Drawing for the job (mm, zero at the part's lowest x, y, z). A direction names the side the tool comes from. Give positions to 0.01 mm unless a question says otherwise; leave off trailing zeros. Order: outer loops, then holes, each group sorted by start corner. A loop starts at its lowest first (then second) coordinate and runs counter-clockwise, first axis right, second up. Notation, with made-up numbers: (25.25, 80) - (36.25, 80) arc R31 cw to (36.25, 119) - close; hole circle Ø9 at (19, -5). An arc over 180 degrees is marked (long way). One line per item, written item: value.
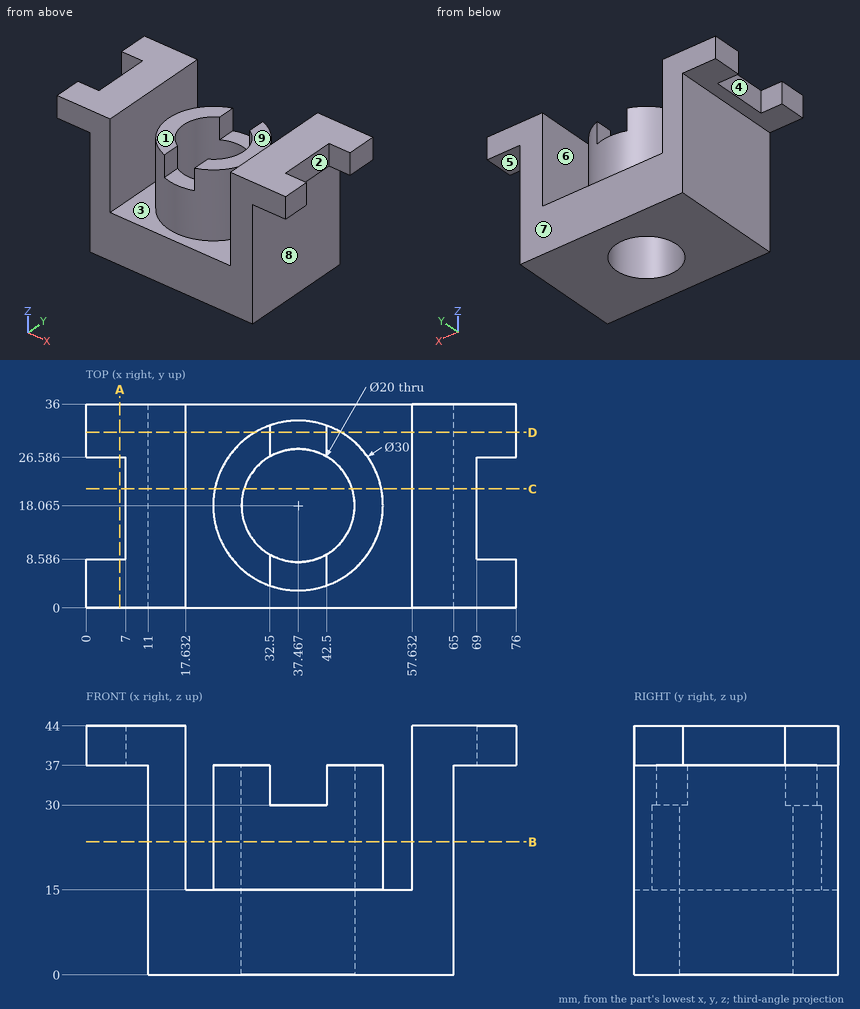
1) Cut at B-B, the plane z = 23.5. Give the cut face in (x, y) (1 decimal).
Outcome:
outline: (11, 0) - (17.6, 0) - (17.6, 36) - (11, 36) - close; circle Ø30 at (37.5, 18.1); (57.6, 0) - (65, 0) - (65, 36) - (57.6, 36) - close; hole circle Ø20 at (37.5, 18.1)
2) Drill centre lines: line 1 along Y through (x, z) = (38, 7); line 2 along X through (y, z) = (13.5, 19.5) (1 decimal); line 3 along X through (y, z) = (21.5, 29.5) (1 decimal). Where is each one in solid material? Low to high. Write a range as from..to.
Outcome:
line 1: y = 0..8.08, 28.05..36
line 2: x = 11..17.6, 23.2..28.6, 46.4..51.8, 57.6..65
line 3: x = 11..17.6, 22.9..28.1, 46.9..52.1, 57.6..65
3) Cut at A-A, the plane x = 6. Give the cut face in (y, z) (1 decimal).
Outcome:
outline: (0, 37) - (8.6, 37) - (8.6, 44) - (0, 44) - close; (26.6, 37) - (36, 37) - (36, 44) - (26.6, 44) - close
4) Which spindle directions (+Z, -Z, +X, -X, +Y, -Y) get a long thin tool onto all of the face, cutting with end or side? Do the marked faces 1, 2, 3, 4 and 5. Say none if no direction does.
Outcome:
face 1: +Z, +Y, -Y
face 2: +Z, -Z, +X
face 3: +Z
face 4: +Z, -Z, -X
face 5: -Z, +X, +Y, -Y
5) Pin check, flat tips, straight feed: pin 1 (12 mm diameter, centred on x = 4.5, y = 14.5, fed in from -Z); pin 2 (11 mm diameter, centred on x = 26, y = 19, fed in from +Z); pin 3 (1.9 mm diameter, centred on x = 35.5, y = 29.5, fed in from +Z). Stop position of each tip, or through.
Outcome:
pin 1: stops at z = 37
pin 2: stops at z = 37
pin 3: stops at z = 30
6) Cut at D-D, the plane y = 31. Give the cut face in (x, z).
Outcome:
outline: (0, 37) - (11, 37) - (11, 0) - (65, 0) - (65, 37) - (76, 37) - (76, 44) - (57.63, 44) - (57.63, 15) - (45.06, 15) - (45.06, 37) - (42.5, 37) - (42.5, 30) - (32.5, 30) - (32.5, 37) - (29.87, 37) - (29.87, 15) - (17.63, 15) - (17.63, 44) - (0, 44) - close
7) Cut at C-C, the plane y = 21. Give the cut face in (x, z).
Outcome:
outline: (7, 37) - (11, 37) - (11, 0) - (27.91, 0) - (27.91, 37) - (22.76, 37) - (22.76, 15) - (17.63, 15) - (17.63, 44) - (7, 44) - close; (47.03, 0) - (65, 0) - (65, 37) - (69, 37) - (69, 44) - (57.63, 44) - (57.63, 15) - (52.18, 15) - (52.18, 37) - (47.03, 37) - close
8) Mould opens along X. For the marked faces 6, 7, 8 and 9 say: released by +X, released by -X, zero draft, split by the parting line, or undercut.
Outcome:
face 6: undercut
face 7: zero draft
face 8: released by +X
face 9: undercut
